```python
from build123d import *

# Parameters (mm, degrees)
F0_W          = 130.1
F0_H          = 2
F1_DEPTH      = 3
F0_W_2        = 142.5
F0_H_2        = 78.4
F0_W_3        = 7
F2_DEPTH      = 3
F2_DEPTH_BACK = 12.7
F3_W          = 5.6
F3_H          = 7.5
F4_DEPTH      = 12.7
F6_DEPTH      = 4.201
F8_DEPTH      = 4.201
F9_DEPTH      = 2
F10_DEPTH     = 2


with BuildPart() as f1:
    # F0 (on Front) → F1 (new body)
    with BuildSketch(Plane.XZ):
        Polygon((67.05, 35), (65.05, 35), (65.05, 33), (65.05, -33), (65.05, -35), (67.05, -35), align=None)
        with Locations((0, 34)):
            Rectangle(F0_W, F0_H)
        Polygon((-65.05, 35), (-67.05, 35), (-67.05, -35), (-65.05, -35), (-65.05, -33), (-65.05, 33), align=None)
        with Locations((0, -34)):
            Rectangle(F0_W, F0_H)
    extrude(amount=-F1_DEPTH)

    # F0 (on Front) → F2 (join, two sides)
    with BuildSketch(Plane.XZ) as f2_sk:
        Rectangle(F0_W_2, F0_H_2)
        Polygon((-67.05, -35), (-67.05, 35), (-65.05, 35), (65.05, 35), (67.05, 35), (67.05, -35), (65.05, -35), (-65.05, -35), align=None, mode=Mode.SUBTRACT)
        with Locations((-74.75, 0)):
            Rectangle(F0_W_3, F0_H_2)
        with Locations((74.75, 0)):
            Rectangle(F0_W_3, F0_H_2)
    extrude(amount=-F2_DEPTH)
    extrude(f2_sk.sketch, amount=F2_DEPTH_BACK)

    # F3 (on face) → F4 (cut)
    with BuildSketch(Plane.XZ.offset(12.7)):
        with Locations((-75.45, 3.75)):
            Rectangle(F3_W, F3_H)
        with Locations((-69.85, 3.75)):
            Rectangle(F3_W, F3_H)
        with Locations((-69.85, -3.75)):
            Rectangle(F3_W, F3_H)
        with Locations((-75.45, -3.75)):
            Rectangle(F3_W, F3_H)
    extrude(amount=-F4_DEPTH, mode=Mode.SUBTRACT)

    # F5 (on face) → F6 (cut, through all)
    with BuildSketch(Plane(origin=(0, 0, 35), x_dir=(1, 0, 0), z_dir=(0, 0, -1))):
        Polygon((47.55, 3.35), (47.55, 6.35), (47.55, 9.35), (32.55, 9.35), (32.55, 3.35), align=None)
    extrude(amount=-F6_DEPTH, mode=Mode.SUBTRACT)

    # F7 (on face) → F8 (cut, through all)
    with BuildSketch(Plane.XY.offset(-35)):
        Polygon((37.05, -9.35), (37.05, -6.35), (37.05, -3.35), (11.05, -3.35), (11.05, -9.35), align=None)
    extrude(amount=-F8_DEPTH, mode=Mode.SUBTRACT)

    # F9 (cut): a face of the model
    f9_faces = [f1.faces().sort_by_distance(p)[0] for p in [
        (24.05, -3.35, -37.1),
    ]]
    extrude(f9_faces, amount=-F9_DEPTH, mode=Mode.SUBTRACT)

    # F10 (cut): a face of the model
    f10_faces = [f1.faces().sort_by_distance(p)[0] for p in [
        (40.05, -3.35, 37.1),
    ]]
    extrude(f10_faces, amount=-F10_DEPTH, mode=Mode.SUBTRACT)


solid = f1.part
```
Here's how the part is built. I have some questions about the finished solid (model axes, mm). A direction names the side the tool comes from. Give positions to 0.01 mm unless a question says otherwise; leave off trailing zeros. Write each loop counter-clockwise with the first axis right and the second up, starting at its lowest first coordinate (ties: lowest second). Pieces come first, ordered by that corner, then holes. Notation, with made-up numbers: M 70,-26.75 L 89,-26.75 A8 ccw 89,-13.75 Z; hole C 78,60 d4. An arc over 180 degrees is marked long. Put each result on its own line as item: value. Start each with the question number.
Item 1: If we section it at C-C, the plane z = 24.5: Write out the boundary of the cut face in (x, y).
Item 2: Thinking about a two-plate mould opening in Z: for faces 5 (the flat face through (1, -5, 39.2)), 6 (the flat face through (-67.05, -6, -21)), 7 (the flat face through (-78.25, 0.5, -0.5)), which applies, +Z half, -Z half, draft (parallel to the pull), parting line (faces both ways), or undercut?
Item 3: On a 3-axis mill with a long thin cutter (end or side, diameter ignored), from which of +Z, -Z, +X, -X, +Y, -Y can I reach the whole of each face in a straight line? I mean faces 1 (the flat face through (40, -9.35, 37)), 2 (the flat face through (11.05, -5, -37)), 3 (the flat face through (1, -6, -35)), 4 (the flat face through (-73, -6, -7.5)). Say none if no direction works.
Item 4: If we section it at A-A, the plane x = 17: Write out the boundary of the cut face in (y, z), then the cut area to 3 significant figures.
Item 5: I need wall thicknesses on L1, parallel to Z at x = -68, y = -6.75; L2, parallel to X at y = -1.5, z = 23; L3, parallel to Z at x = 6, y = -9.5. Which ranges of each line are inside material? Lowest first, please. Write a range as from..to.
Item 6: If we section it at D-D, the plane x = -2: Write out the boundary of the cut face in (y, z).
Item 7: If we section it at B-B, the plane y = -5: Write out the boundary of the cut face in (x, z).
Values:
1. outline: M -78.25,-12.7 L -67.05,-12.7 L -67.05,0 L -65.05,0 L -65.05,3 L -78.25,3 Z; M 65.05,0 L 67.05,0 L 67.05,-12.7 L 78.25,-12.7 L 78.25,3 L 65.05,3 Z
2. face 5: +Z half
2. face 6: undercut
2. face 7: draft
3. face 1: +Z
3. face 2: -Z
3. face 3: -Y
3. face 4: -X, -Y
4. outline: M -12.7,-39.2 L -9.35,-39.2 L -9.35,-35 L -12.7,-35 Z; M -12.7,35 L 0,35 L 0,33 L 3,33 L 3,39.2 L -12.7,39.2 Z; M -1.35,-39.2 L 3,-39.2 L 3,-33 L 0,-33 L 0,-35 L -1.35,-35 Z
4. area: 110 mm²
5. L1: -39.2..-7.5, 7.5..39.2
5. L2: -78.25..-67.05, 67.05..78.25
5. L3: -39.2..-35, 35..39.2
6. outline: M -12.7,-39.2 L 3,-39.2 L 3,-33 L 0,-33 L 0,-35 L -12.7,-35 Z; M -12.7,35 L 0,35 L 0,33 L 3,33 L 3,39.2 L -12.7,39.2 Z
7. outline: M -78.25,-39.2 L 11.05,-39.2 L 11.05,-35 L -67.05,-35 L -67.05,-7.5 L -78.25,-7.5 Z; M -78.25,7.5 L -67.05,7.5 L -67.05,35 L 32.55,35 L 32.55,39.2 L -78.25,39.2 Z; M 37.05,-39.2 L 78.25,-39.2 L 78.25,39.2 L 47.55,39.2 L 47.55,35 L 67.05,35 L 67.05,-35 L 37.05,-35 Z
